Autodesk Inventor part; units mm, degrees
ref_plane "YZ Plane" through (0, 0, 0) normal (1, 0, 0) x (0, 1, 0)
ref_plane "XZ Plane" through (0, 0, 0) normal (0, 1, 0) x (-1, 0, 0)
ref_plane "XY Plane" through (0, 0, 0) normal (0, 0, 1) x (1, 0, 0)
sketch "Sketch1" plane through (0, 0, 0) normal (1, 0, 0) x (0, 1, 0)
  circle A0 centre (0, 0) radius 2.5
  dimension "d0" = 5
extrude "Extrusion1" add sketch "Sketch1" along normal blind 101.6
sketch "Sketch2" plane through (0, 0, 0) normal (-1, 0, 0) x (0, 0, 1)
  point P0 (0, 0)
sketch "Sketch3" plane through (0, 0, 0) normal (-1, 0, 0) x (0, 0, 1)
  circle A0 centre (0, 0) radius 2.5
  dimension "d3" = 5
extrude "Extrusion2" add sketch "Sketch3" along normal blind 50.8
sketch "Sketch4" plane through (101.6, 0, 0) normal (1, 0, 0) x (0, 0, -1)
  point P0 (0, 0)
sketch "Sketch5" plane through (-50.8, 0, 0) normal (-1, 0, 0) x (0, 0, 1)
  circle A0 centre (0, 0) radius 5
  dimension "d6" = 10
extrude "Extrusion3" add sketch "Sketch5" against normal blind 10
properties part number "cylindre plateform"
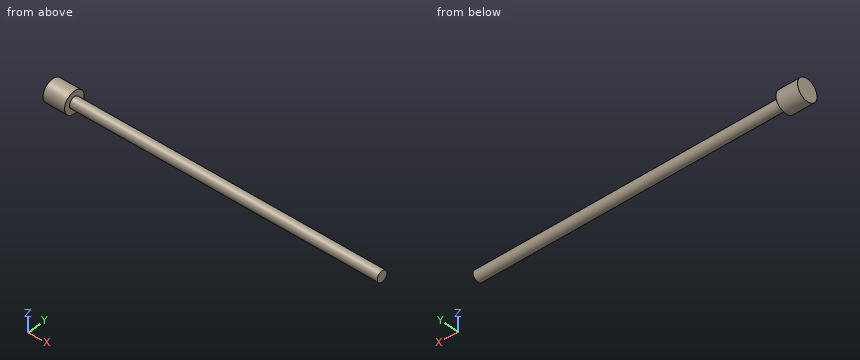
Verification items for the finished model (mm, model axes). Give positions to 0.01 mm unless a question says otherwise; leave off trailing zeros. Loops run counter-clockwise (first coordinate to the right, second up) from the corner with the lowest first, then second, coordinate; pieces in that order, holes last.
1) Depth check by flat-ended pin: pin 1 Ø1.5 at (y, z) = (3, 2) entering from +X; pin 2 Ø3 at (x, z) = (78.5, 3.5) entering from -Y; pin 3 Ø5 at (x, y) = (-26, -1.5) entering from -Z. Enter the tip coordinate at first touch or a pass-through.
2) Sectioned sample at A-A, the plane x = -8. Enter the section's corners in (y, z), then the cut area to 3 significant figures.
3) Thickness scan on line 1 along X through (y, z) = (-3, 3.75); line 2 along Z through (x, y) = (18, -0.25); line 3 along Y through (x, z) = (-43.5, 0.25). Record the ranges inside material, lowest first.
Answers:
1. pin 1: stops at x = -40.8
1. pin 2: stops at y = -1.5
1. pin 3: stops at z = -2.5
2. outline: circle Ø5 at (0, 0)
2. area: 19.6 mm2
3. line 1: x = -50.8 to -40.8
3. line 2: z = -2.49 to 2.49
3. line 3: y = -4.99 to 4.99
